```python
from build123d import *

# Parameters (mm, degrees)
SKETCH1_W           = 240
SKETCH1_H           = 45
SKETCH1_R           = 1.5
SKETCH1_W_2         = 5
SKETCH1_H_2         = 10
BOSS_EXTRUDE1_DEPTH = 5
CUT_EXTRUDE1_DEPTH  = 5
FILLET1_R           = 1


with BuildPart() as part:
    # Sketch1 → Boss-Extrude1 (new body)
    with BuildSketch(Plane.XY):
        with Locations((34.186746988, 0)):
            Rectangle(SKETCH1_W, SKETCH1_H)
        with Locations((-78.313253012, 0)):
            Circle(SKETCH1_R, mode=Mode.SUBTRACT)
        with Locations(Location((146.686746988, 0, 0), (0, 0, 180))):
            Circle(SKETCH1_R, mode=Mode.SUBTRACT)
        with Locations((-78.313253012, -15)):
            Rectangle(SKETCH1_W_2, SKETCH1_H_2, mode=Mode.SUBTRACT)
        with Locations((-78.313253012, 15)):
            Rectangle(SKETCH1_W_2, SKETCH1_H_2, mode=Mode.SUBTRACT)
        with Locations((146.686746988, -15)):
            Rectangle(SKETCH1_W_2, SKETCH1_H_2, mode=Mode.SUBTRACT)
        with Locations((146.686746988, 15)):
            Rectangle(SKETCH1_W_2, SKETCH1_H_2, mode=Mode.SUBTRACT)
    extrude(amount=BOSS_EXTRUDE1_DEPTH)

    # Sketch2 → Cut-Extrude1 (cut)
    with BuildSketch(Plane.XY.offset(5)):
        with BuildLine():
            Line((-71.313253012, 22.5), (-60.313253012, 22.5))
            Line((-60.313253012, 22.5), (-61.563253012, 10))
            ThreePointArc((-61.563253012, 10), (-65.813253012, 5.75), (-70.063253012, 10))
            Line((-70.063253012, 10), (-71.313253012, 22.5))
        make_face()
        with BuildLine():
            Line((-46.313253012, 22.5), (-35.313253012, 22.5))
            Line((-35.313253012, 22.5), (-36.563253012, 10))
            ThreePointArc((-36.563253012, 10), (-40.813253012, 5.75), (-45.063253012, 10))
            Line((-45.063253012, 10), (-46.313253012, 22.5))
        make_face()
        with BuildLine():
            Line((-21.313253012, 22.5), (-10.313253012, 22.5))
            Line((-10.313253012, 22.5), (-11.563253012, 10))
            ThreePointArc((-11.563253012, 10), (-15.813253012, 5.75), (-20.063253012, 10))
            Line((-20.063253012, 10), (-21.313253012, 22.5))
        make_face()
        with BuildLine():
            Line((3.686746988, 22.5), (14.686746988, 22.5))
            Line((14.686746988, 22.5), (13.436746988, 10))
            ThreePointArc((13.436746988, 10), (9.186746988, 5.75), (4.936746988, 10))
            Line((4.936746988, 10), (3.686746988, 22.5))
        make_face()
        with BuildLine():
            Line((28.686746988, 22.5), (39.686746988, 22.5))
            Line((39.686746988, 22.5), (38.436746988, 10))
            ThreePointArc((38.436746988, 10), (34.186746988, 5.75), (29.936746988, 10))
            Line((29.936746988, 10), (28.686746988, 22.5))
        make_face()
        with BuildLine():
            Line((53.686746988, 22.5), (64.686746988, 22.5))
            Line((64.686746988, 22.5), (63.436746988, 10))
            ThreePointArc((63.436746988, 10), (59.186746988, 5.75), (54.936746988, 10))
            Line((54.936746988, 10), (53.686746988, 22.5))
        make_face()
        with BuildLine():
            Line((78.686746988, 22.5), (89.686746988, 22.5))
            Line((89.686746988, 22.5), (88.436746988, 10))
            ThreePointArc((88.436746988, 10), (84.186746988, 5.75), (79.936746988, 10))
            Line((79.936746988, 10), (78.686746988, 22.5))
        make_face()
        with BuildLine():
            Line((103.686746988, 22.5), (114.686746988, 22.5))
            Line((114.686746988, 22.5), (113.436746988, 10))
            ThreePointArc((113.436746988, 10), (109.186746988, 5.75), (104.936746988, 10))
            Line((104.936746988, 10), (103.686746988, 22.5))
        make_face()
        with BuildLine():
            Line((128.686746988, 22.5), (139.686746988, 22.5))
            Line((139.686746988, 22.5), (138.436746988, 10))
            ThreePointArc((138.436746988, 10), (134.186746988, 5.75), (129.936746988, 10))
            Line((129.936746988, 10), (128.686746988, 22.5))
        make_face()
        with BuildLine():
            Line((139.686746988, -22.5), (138.436746988, -10))
            ThreePointArc((138.436746988, -10), (134.186746988, -5.75), (129.936746988, -10))
            Line((129.936746988, -10), (128.686746988, -22.5))
            Line((128.686746988, -22.5), (139.686746988, -22.5))
        make_face()
        with BuildLine():
            Line((114.686746988, -22.5), (113.436746988, -10))
            ThreePointArc((113.436746988, -10), (109.186746988, -5.75), (104.936746988, -10))
            Line((104.936746988, -10), (103.686746988, -22.5))
            Line((103.686746988, -22.5), (114.686746988, -22.5))
        make_face()
        with BuildLine():
            Line((89.686746988, -22.5), (88.436746988, -10))
            ThreePointArc((88.436746988, -10), (84.186746988, -5.75), (79.936746988, -10))
            Line((79.936746988, -10), (78.686746988, -22.5))
            Line((78.686746988, -22.5), (89.686746988, -22.5))
        make_face()
        with BuildLine():
            Line((64.686746988, -22.5), (63.436746988, -10))
            ThreePointArc((63.436746988, -10), (59.186746988, -5.75), (54.936746988, -10))
            Line((54.936746988, -10), (53.686746988, -22.5))
            Line((53.686746988, -22.5), (64.686746988, -22.5))
        make_face()
        with BuildLine():
            Line((39.686746988, -22.5), (38.436746988, -10))
            ThreePointArc((38.436746988, -10), (34.186746988, -5.75), (29.936746988, -10))
            Line((29.936746988, -10), (28.686746988, -22.5))
            Line((28.686746988, -22.5), (39.686746988, -22.5))
        make_face()
        with BuildLine():
            Line((14.686746988, -22.5), (13.436746988, -10))
            ThreePointArc((13.436746988, -10), (9.186746988, -5.75), (4.936746988, -10))
            Line((4.936746988, -10), (3.686746988, -22.5))
            Line((3.686746988, -22.5), (14.686746988, -22.5))
        make_face()
        with BuildLine():
            Line((-10.313253012, -22.5), (-11.563253012, -10))
            ThreePointArc((-11.563253012, -10), (-15.813253012, -5.75), (-20.063253012, -10))
            Line((-20.063253012, -10), (-21.313253012, -22.5))
            Line((-21.313253012, -22.5), (-10.313253012, -22.5))
        make_face()
        with BuildLine():
            Line((-35.313253012, -22.5), (-36.563253012, -10))
            ThreePointArc((-36.563253012, -10), (-40.813253012, -5.75), (-45.063253012, -10))
            Line((-45.063253012, -10), (-46.313253012, -22.5))
            Line((-46.313253012, -22.5), (-35.313253012, -22.5))
        make_face()
        with BuildLine():
            Line((-60.313253012, -22.5), (-61.563253012, -10))
            ThreePointArc((-61.563253012, -10), (-65.813253012, -5.75), (-70.063253012, -10))
            Line((-70.063253012, -10), (-71.313253012, -22.5))
            Line((-71.313253012, -22.5), (-60.313253012, -22.5))
        make_face()
    extrude(amount=-CUT_EXTRUDE1_DEPTH, mode=Mode.SUBTRACT)

    # Fillet1
    fillet1_edges = [part.edges().sort_by_distance(p)[0] for p in [
        (-60.313253012, -22.5, 2.5),
        (-71.313253012, -22.5, 2.5),
        (-35.313253012, -22.5, 2.5),
        (-46.313253012, -22.5, 2.5),
        (-10.313253012, -22.5, 2.5),
        (-21.313253012, -22.5, 2.5),
        (14.686746988, -22.5, 2.5),
        (3.686746988, -22.5, 2.5),
        (39.686746988, -22.5, 2.5),
        (28.686746988, -22.5, 2.5),
        (64.686746988, -22.5, 2.5),
        (53.686746988, -22.5, 2.5),
        (89.686746988, -22.5, 2.5),
        (78.686746988, -22.5, 2.5),
        (114.686746988, -22.5, 2.5),
        (103.686746988, -22.5, 2.5),
        (139.686746988, -22.5, 2.5),
        (128.686746988, -22.5, 2.5),
        (128.686746988, 22.5, 2.5),
        (139.686746988, 22.5, 2.5),
        (103.686746988, 22.5, 2.5),
        (114.686746988, 22.5, 2.5),
        (78.686746988, 22.5, 2.5),
        (89.686746988, 22.5, 2.5),
        (53.686746988, 22.5, 2.5),
        (64.686746988, 22.5, 2.5),
        (28.686746988, 22.5, 2.5),
        (39.686746988, 22.5, 2.5),
        (3.686746988, 22.5, 2.5),
        (14.686746988, 22.5, 2.5),
        (-21.313253012, 22.5, 2.5),
        (-10.313253012, 22.5, 2.5),
        (-46.313253012, 22.5, 2.5),
        (-35.313253012, 22.5, 2.5),
        (-71.313253012, 22.5, 2.5),
        (-60.313253012, 22.5, 2.5),
        (-85.813253012, 22.5, 2.5),
        (154.186746988, 22.5, 2.5),
        (154.186746988, -22.5, 2.5),
        (-85.813253012, -22.5, 2.5),
    ]]
    fillet(fillet1_edges, radius=FILLET1_R)


solid = part.part
```
Input: part model. Units: mm. Frame: model coordinates. A direction names the side the tool comes from. Coordinates: 2 decimals unless noted, no trailing zeros. Loops run counter-clockwise (first coordinate to the right, second up) from the corner with the lowest first, then second, coordinate; pieces in that order, holes last. Notation, with made-up numbers: M 73.5,45 L 77.5,45 A7 ccw 77.5,58 Z; hole C 61.5,7.25 d8. An arc over 180 degrees is marked long. Answer in a Markdown table with one row per item.
1. Draft query along X for faces 1 (the flat face through (-78, 20, 2)), 2 (the flat face through (22, -22.5, 2)). Return one class per face: pulls with the +X half, pulls with the -X half, needs draft (parallel to the pull), parting line crosses it, or undercut.
Response:
| item | result |
|---|---|
| face 1 | undercut |
| face 2 | needs draft |
2. Material intervals for line 1 (Y direction, x = -72, z = 1.9); line 2 (Y direction, x = 59.5, z = 4.8), sorted ascending.
Response:
| item | result |
|---|---|
| line 1 | y = -22.48 to 22.48 |
| line 2 | y = -5.76 to 5.76 |
3. Reachability of faces 3 (the flat face through (-80.813, -15, 2)), 4 (the flat face through (-60.975, -15.881, 2.535)), 5 (the flat face through (29.365, 15.719, 2.535)), 6 (the flat face through (6, 0, 5)) from +Z, -Z, +X, -X, +Y, -Y: full face, straight path, thin tool, end or side. Return the list, or none.
Response:
| item | result |
|---|---|
| face 3 | +Z, -Z |
| face 4 | +Z, -Z, -Y |
| face 5 | +Z, -Z, +Y |
| face 6 | +Z, +X, -X, +Y, -Y |
4. First-contact query: pin 1 (4 mm diameter, centred on x = 146.69, y = 0, fed in from -Z). Flat tip, straight axial feed; report the tip coordinate or a pass-through.
Response:
| item | result |
|---|---|
| pin 1 | stops at z = 0 |
5. Section C-C, the plane x = -40. Output: boundary loops of the cut face in (y, z).
Response:
| item | result |
|---|---|
| outline | M -5.83,0 L 5.83,0 L 5.83,5 L -5.83,5 Z |
6. Section A-A, the plane z = 1.55. Count the separate pieces of the cut face and the enclosed holes in it, then the cut area to 3 significant figures.
Response:
| item | result |
|---|---|
| separate pieces | 1 |
| enclosed holes | 6 |
| area | 7,870 mm2 |
